Can you work these out from the drawing? Everything is in mm from the part's minimum corner. A direction names the side the tool comes from. Coordinates: 2 decimals unless noted, no trailing zeros. Order: outer loops, then holes, each group sorted by start corner. A loop starts at its lowest first (then second) coordinate and runs counter-clockwise, first axis right, second up. Notation, with made-up numbers: M -22,-16 L 35,-16 A9 cw 35,1 Z; hole C 70,-32 d9. An arc over 180 degrees is marked long. One line per question, with ' | ' between items. Start each with the question number.
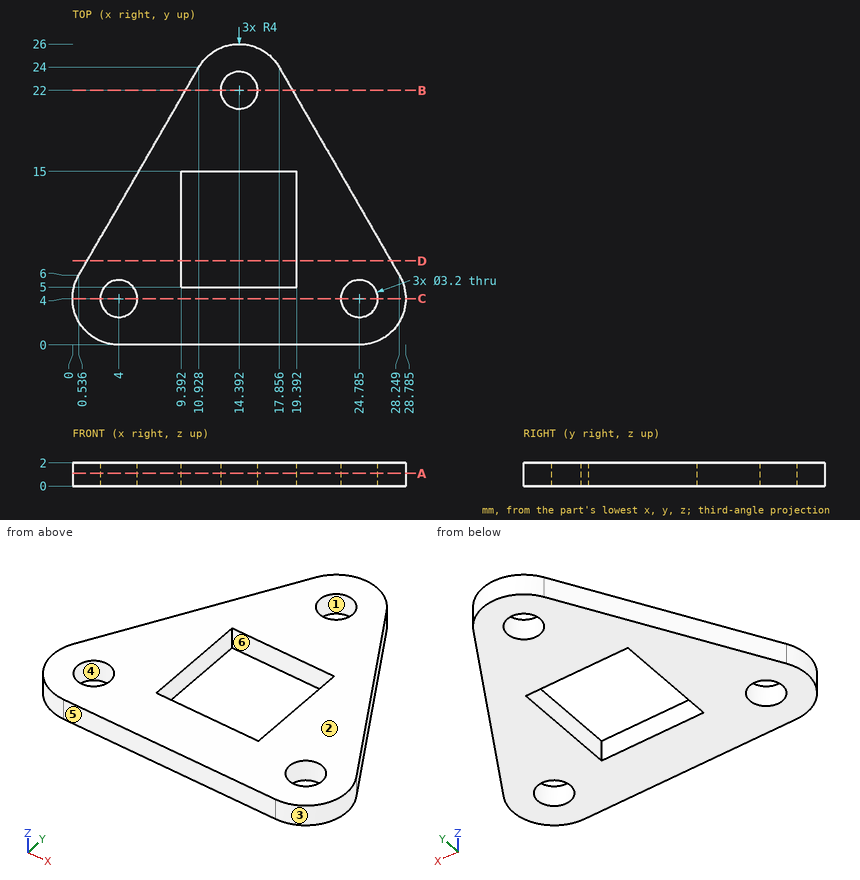
(1) We'd pull the mould along Y, two halves only. Please class the marked faces 1, 2, 3 and 4: +Y half, -Y half, draft (parallel to the pull), parting line (faces both ways), or undercut.
(2) Imagine slicing it at A-A, the plane z = 1.1. Write out the boundary of the cut face in (x, y) (1 decimal).
(3) On a 3-axis mill with a long thin cutter (end or side, diameter ignored), from which of +Z, -Z, +X, -X, +Y, -Y can I reach the whole of each face in a straight line? I mean the marked faces 5 and 6. Say none if no direction works.
(4) If I drill on line 1 along X through (y, z) = (14.5, 1.85) (1 decimal); line 2 along Y through (x, z) = (1.5, 0.85) (1 decimal); line 3 along Y through (x, z) = (8.25, 0.15), over which ranges is the centre line in solid material (lowest first)? Write a range as from..to.
(5) Imagine slicing it at C-C, the plane y = 4. Write out the boundary of the cut face in (x, z) (1 decimal).
(6) For P1, Ø0.6, axis at x = 13, z = 1.5, coming from the +Y side; P2, Ø0.6, axis at y = 9, z = 1, coming from the +X side, each with a flat end and sliding along its axis, tell me the tip position at first contact or that it passes through.
(7) Imagine slicing it at B-B, the plane y = 22. Write out the boundary of the cut face in (x, z).
(8) Imagine slicing it at D-D, the plane y = 7.25. Write out the boundary of the cut face in (x, z).
Answers:
1) face 1: undercut | face 2: draft | face 3: parting line | face 4: undercut
2) outline: M 0.5,6 A4 ccw 4,0 L 24.8,0 A4 ccw 28.2,6 L 17.9,24 A4 ccw 10.9,24 Z; hole C 4,4 d3.2; hole M 9.4,5 L 19.4,5 L 19.4,15 L 9.4,15 Z; hole C 14.4,22 d3.2; hole C 24.8,4 d3.2
3) face 5: +Z, -Z, +X, -X, -Y | face 6: +Z, -Z
4) line 1: 5.4..9.4, 19.4..23.3 | line 2: 0.9..7.7 | line 3: 0..19.36
5) outline: M 0,0 L 2.4,0 L 2.4,2 L 0,2 Z; M 5.6,0 L 23.2,0 L 23.2,2 L 5.6,2 Z; M 26.4,0 L 28.8,0 L 28.8,2 L 26.4,2 Z
6) P1: y = 25.85 | P2: x = 26.69
7) outline: M 9.77,0 L 12.79,0 L 12.79,2 L 9.77,2 Z; M 15.99,0 L 19.01,0 L 19.01,2 L 15.99,2 Z
8) outline: M 1.26,0 L 9.39,0 L 9.39,2 L 1.26,2 Z; M 19.39,0 L 27.53,0 L 27.53,2 L 19.39,2 Z
